Geometry check sheet. Reference: the model listing, model coordinates, mm. Face numbers are marked on the shaded views. Coordinates: 2 decimals unless noted, no trailing zeros. Loops run counter-clockwise (first coordinate to the right, second up) from the corner with the lowest first, then second, coordinate; pieces in that order, holes last. Notation, with made-up numbers: (-34, 49.5) -> (19, 49.5) arc R9 ccw to (19, 65.5) -> close; hole circle Ø9 at (74, -1). An arc over 180 degrees is marked (long way). Answer as a JSON object with one key per item and string values.
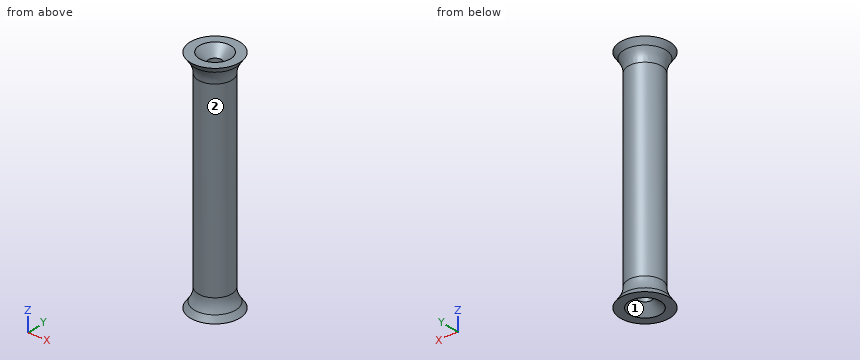
from build123d import *

# Parameters (mm, degrees)
F2_R     = 5
F3_SIZE2 = 2
F3_SIZE  = 2


with BuildPart() as f1:
    # F0 (on Front) → F1 (revolve)
    with BuildSketch(Plane.XZ):
        Polygon((-13.5647695723, 9.2907883497), (-17.5647695723, 9.2907883497), (-15.8147693879, 6.7407885124), (-15.8147693879, -15.7092116503), (-13.5647695723, -15.7092116503), align=None)
        Polygon((-13.5647695723, -40.7092116503), (-13.5647695723, -15.7092116503), (-15.8147693879, -15.7092116503), (-15.8147693879, -38.159211813), (-17.5647695723, -40.7092116503), align=None)
    revolve(axis=Axis((-12.1147695723, 0, -13.6592119893), (0, 0, -1)))

    # F2
    f2_edges = [f1.edges().sort_by_distance(p)[0] for p in [
        (-8.41477, 0, 6.740789),
        (-8.41477, 0, -38.159212),
    ]]
    fillet(f2_edges, radius=F2_R)

    # F3
    f3_edges = [f1.edges().sort_by_distance(p)[0] for p in [
        (-10.66477, 0, 9.290788),
        (-10.66477, 0, -40.709212),
    ]]
    chamfer(f3_edges, length=F3_SIZE, length2=F3_SIZE2)


solid = f1.part
1. Mould release check, pull along Y, two halves, no side actions. Record for the marked faces 1 and 2: released by +Y, released by -Y, zero draft, split by the parting line, or undercut.
Evaluation:
{"face 1": "undercut", "face 2": "split by the parting line"}
2. Section check A-A, the plane z = 4.5. Record the boundary of the cut face in (x, y).
Evaluation:
{"outline": "circle Ø7.4 at (-12.11, 0); hole circle Ø2.9 at (-12.11, 0)"}
3. Thickness scan on probe 1 along Y at (x, z) = (-13, -24); probe 2 along Z at (x, y) = (-15.75, -3.75); probe 3 along Y at (x, z) = (-12.5, -38). Record the ranges inside material, lowest first. Write a range as from..to.
Evaluation:
{"probe 1": "y = -3.59..-1.15, 1.15..3.59", "probe 2": "z = -40.71..-40.38, 8.96..9.29", "probe 3": "y = -3.88..-1.4, 1.4..3.88"}
4. Depth check by flat-ended pin: P1, Ø4, axis at x = -12.11, y = 0, coming from the +Z side; P2, Ø2, axis at y = 3, z = -31.5, coming from the +X side; P3, Ø4, axis at x = -9.5, z = -28, coming from the +Y side. Enter the tip coordinate at first touch or a pass-through.
Evaluation:
{"P1": "stops at z = 7.85", "P2": "stops at x = -9", "P3": "stops at y = 3.65"}
